```python
from build123d import *

# Parameters (mm, degrees)
EXTRUDE_1_DEPTH     = 240
SHELL_1_T           = 1
CUT_EXTRUDE_1_DEPTH = 10
SKETCH_3_R          = 3.0000000000000018
SKETCH_3_R_2        = 3.000000000000008
CUT_EXTRUDE_2_DEPTH = 10
CUT_EXTRUDE_START   = -8
SKETCH_6_R          = 3.0000000000000018
SKETCH_6_R_2        = 3.000000000000008
CUT_EXTRUDE_4_DEPTH = 8


with BuildPart() as part:
    # 草图1 → 凸台-拉伸1 (new body)
    with BuildSketch(Plane.XY):
        with BuildLine():
            Line((-59.31594071221176, -68.02781651157832), (-59.9536030402972, -73.74672011248332))
            ThreePointArc((-59.9536030402972, -73.74672011248332), (-57.826283597547295, -81.098805241968), (-51.12333234290943, -84.79327248916888))
            Line((-51.12333234290943, -84.79327248916888), (48.260783027457215, -95.87468088565784))
            ThreePointArc((48.260783027457215, -95.87468088565784), (70.3170384159113, -89.49272255740806), (81.40044015751394, -69.38386879349436))
            Line((81.40044015751394, -69.38386879349436), (88.61365635961639, -4.691811108090497))
            Line((88.61365635961639, -4.691811108090497), (84.83705997568286, -4.270717589039598))
            Line((84.83705997568286, -4.270717589039598), (89.4084892426148, 36.72835377657124))
            ThreePointArc((89.4084892426148, 36.72835377657124), (87.266542040995, 44.098694219102335), (80.53170892213036, 47.77998188979318))
            Line((80.53170892213036, 47.77998188979318), (-41.90893576965496, 60.852539535143315))
            Line((-41.90893576965496, 60.852539535143315), (-55.71014158484277, -68.41279502152355))
            Line((-55.71014158484277, -68.41279502152355), (-59.190362130599055, -68.04122409572891))
            Line((-59.190362130599055, -68.04122409572891), (-59.31594071221176, -68.02781651157832))
        make_face()
    extrude(amount=EXTRUDE_1_DEPTH)

    # 抽壳1
    shell_1_openings = [part.faces().sort_by_distance(p)[0] for p in [
        (-48.809538677, -3.780127743, 120),
        (19.311386576, 54.316260712, 120),
        (87.266542041, 44.098694219, 120),
        (87.122774609, 16.228818094, 120),
        (86.725358168, -4.481264349, 120),
        (-57.513041149, -68.220305767, 120),
    ]]
    offset(amount=SHELL_1_T, openings=shell_1_openings, kind=Kind.INTERSECTION)

    # 草图2 → 切除-拉伸1 (cut)
    with BuildSketch(Plane(origin=(0, 0, -1), x_dir=(-1, 0, 0), z_dir=(0, 0, -1))):
        with BuildLine():
            Line((47.084151642276574, 12.380252393304023), (24.71130527686598, 9.991582155982451))
            ThreePointArc((24.71130527686598, 9.991582155982451), (6.908463771051354, 15.233207386949033), (-1.9736574368444393, 31.528106085354896))
            Line((-1.9736574368444393, 31.528106085354896), (-4.574653917520899, 55.88964990582092))
            Line((-4.574653917520899, 55.88964990582092), (41.90893576965496, 60.852539535143315))
            Line((41.90893576965496, 60.852539535143315), (47.084151642276574, 12.380252393304023))
        make_face()
    extrude(amount=-CUT_EXTRUDE_1_DEPTH, mode=Mode.SUBTRACT)

    # 草图3 → 切除-拉伸2 (cut)
    with BuildSketch(Plane(origin=(0, 0, -1), x_dir=(-1, 0, 0), z_dir=(0, 0, -1))):
        with Locations((-25.52734826155789, 49.12702905294972)):
            Circle(SKETCH_3_R)
        with Locations((-82.20224799889411, 12.905547308509762)):
            Circle(SKETCH_3_R_2)
        with Locations((49.590043926063395, -53.47812379490241)):
            Circle(SKETCH_3_R)
    extrude(amount=-CUT_EXTRUDE_2_DEPTH, mode=Mode.SUBTRACT)

    # 草图6 → 切除-拉伸4 (cut)
    with BuildSketch(Plane.XY.offset(241).offset(CUT_EXTRUDE_START)):
        with Locations(Location((25.52734826155789, 49.12702905294972, 0), (0, 0, 180))):
            Circle(SKETCH_6_R)
        with Locations(Location((82.20224799889411, 12.905547308509762, 0), (0, 0, 180))):
            Circle(SKETCH_6_R_2)
        with Locations(Location((-49.590043926063395, -53.47812379490241, 0), (0, 0, 180))):
            Circle(SKETCH_6_R)
    extrude(amount=CUT_EXTRUDE_4_DEPTH, mode=Mode.SUBTRACT)


solid = part.part
```
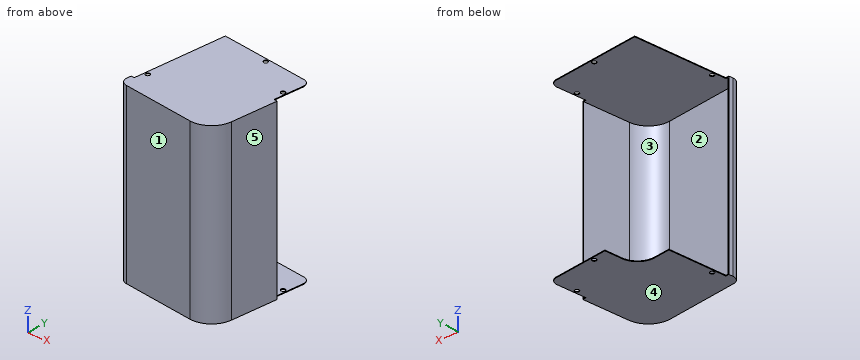
Input: part model. Units: mm. Frame: model coordinates. Face numbers are marked on the shaded views. A direction names the side the tool comes from. Give positions to 0.01 mm unless a question says otherwise; leave off trailing zeros. Order: outer loops, then holes, each group sorted by start corner. A loop starts at its lowest first (then second) coordinate and runs counter-clockwise, first axis right, second up. Notation, with made-up numbers: (69.25, 81.5) - (98.25, 81.5) arc R21 cw to (98.25, 101.5) - close; hole circle Ø9 at (-35, -10). An arc over 180 degrees is marked (long way). Use a Markdown table: item, result.
(1) Section query D-D (x = -16). Output: boundary loops of the cut face in (y, z), then the cut area to 3 significant figures.
Computed values:
| item | result |
|---|---|
| outline | (-89.72, -1) - (10.64, -1) - (10.64, 0) - (-88.71, 0) - (-88.71, 240) - (58.09, 240) - (58.09, 241) - (-89.72, 241) - close |
| area | 490 mm2 |
(2) Access query for the marked faces 1 and 2. Directions: +Z, -Z, +X, -X, +Y, -Y. A direction counts if a zero-diameter tool reaches every point of the face in a straight line with its end or side. Return the directions, or none.
Computed values:
| item | result |
|---|---|
| face 1 | +Z, -Z, -X, -Y |
| face 2 | +Y |
(3) Line query: line 1 (Z direction, x = 21.5, y = -80); line 2 (Z direction, x = -29.5, y = 54.5); line 3 (X direction, y = -81, z = 21). Output: solid intervals per line, ascending. Write a range as from..to.
Computed values:
| item | result |
|---|---|
| line 1 | z = -1..0, 240..241 |
| line 2 | z = 240..241 |
| line 3 | x = -59.14..-57.9, 77.6..78.75 |
(4) Section query A-A (z = 16). Output: boundary loops of the cut face in (x, y), then the cut area to 3 significant figures.
Computed values:
| item | result |
|---|---|
| outline | (-60.95, -73.64) arc R11 ccw to (-51.23, -85.79) - (48.15, -96.87) arc R31 ccw to (82.39, -69.49) - (89.61, -4.8) - (88.61, -4.69) - (81.4, -69.38) arc R30 cw to (48.26, -95.87) - (-51.12, -84.79) arc R10 cw to (-59.95, -73.75) - (-59.32, -68.03) - (-60.31, -67.92) - close |
| area | 235 mm2 |
(5) Section query B-B (y = 26). Output: boundary loops of the cut face in (x, z), then the cut area to 3 significant figures.
Computed values:
| item | result |
|---|---|
| outline | (-45.63, 240) - (88.21, 240) - (88.21, 241) - (-45.63, 241) - close; (0.72, -1) - (88.21, -1) - (88.21, 0) - (0.72, 0) - close |
| area | 221 mm2 |
(6) Draft query along Z for the marked faces 3, 4 and 5. Return one class per face: released by +Z, released by -Z, zero draft, split by the parting line, or undercut.
Computed values:
| item | result |
|---|---|
| face 3 | undercut |
| face 4 | released by -Z |
| face 5 | zero draft |
(7) Section query C-C (y = -79). Output: boundary loops of the cut face in (x, z).
Computed values:
| item | result |
|---|---|
| outline | (-60.2, -1) - (79.76, -1) - (79.76, 241) - (-60.2, 241) - close; hole (-59.12, 0) - (78.65, 0) - (78.65, 240) - (-59.12, 240) - close |
(8) Pin query (flat end, axial travel): pin 1 (8 mm diameter, centred on y = -68, z = 195.5, fed in from +X); pin 2 (12 mm diameter, centred on x = 29, z = 131.5, fed in from +Y); pin 3 (5.5 mm diameter, centred on x = 25.53, y = 49.13, fed in from +Z); pin 4 (4 mm diameter, centred on x = 40.5, z = 202.5, fed in from -Y). Return the tip coordinate at first contact, or that it passes through.
Computed values:
| item | result |
|---|---|
| pin 1 | stops at x = 83.01 |
| pin 2 | stops at y = -93.06 |
| pin 3 | passes through |
| pin 4 | stops at y = -96.24 |
